Work out the finished part from the listing and answer in its coordinate system (mm). Face numbers are marked on the shaded views. Coordinates: 2 decimals unless noted, no trailing zeros. Order: outer loops, then holes, each group sorted by start corner. A loop starts at its lowest first (then second) coordinate and runs counter-clockwise, first axis right, second up. Notation, with made-up numbers: M 32,4 L 46,4 A21 ccw 46,31 Z; hole C -9,73.25 d10. An arc over 180 degrees is marked long. Answer in a Markdown table with one row per item. Add a question column.
Item 1: The part is cut by section A-A (z = 0). Write down the section's boundary in (x, y), then the cut area to 3 significant figures.
Item 2: The mould has two halves that part along Z. Classify the marked faces 1, 2 and 3: released by +Z, released by -Z, zero draft, split by the parting line, or undercut.
Item 3: Consider line 1 (Y direction, x = 5, z = 0); line 2 (Y direction, x = 2.25, z = -13.5); line 3 (Y direction, x = 5.75, z = 25). Determine where each line is inside the solid, lowest interval first. Write a range as from..to.
Item 4: Flat-ended cylindrical pins translate along their axes: pin 1 Ø3 at (x, y) = (1.5, 156) entering from -Z; pin 2 Ø2 at (x, z) = (7.5, 23) entering from +Y; pin 3 Ø5 at (x, y) = (2, -8.5) entering from +Z. Find the tip coordinate at first contact, or state that the pin passes through.
Item 5: The part is cut by section C-C (x = 2). Write down the section's boundary in (y, z).
Item 6: The part is cut by section B-B (y = 142.5). Write down the section's boundary in (x, z).
Item 7: The part is cut by section D-D (z = -20.5). Write down the section's boundary in (x, y), then the cut area to 3 significant figures.
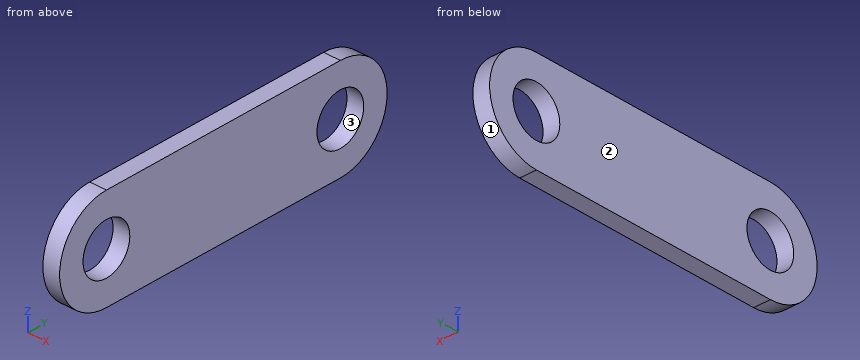
from build123d import *

# Parameters (mm, degrees)
SKETCH1_R           = 15
BOSS_EXTRUDE1_DEPTH = 10


with BuildPart() as part:
    # Sketch1 → Boss-Extrude1 (new body)
    with BuildSketch(Plane.YZ):
        with BuildLine():
            Line((0, 30), (150, 30))
            ThreePointArc((150, 30), (180, 0), (150, -30))
            Line((150, -30), (0, -30))
            ThreePointArc((0, -30), (-30, 0), (0, 30))
        make_face()
        with Locations(Location((0, 0, 0), (0, 0, 270))):
            Circle(SKETCH1_R, mode=Mode.SUBTRACT)
        with Locations(Location((150, 0, 0), (0, 0, 270))):
            Circle(SKETCH1_R, mode=Mode.SUBTRACT)
    extrude(amount=BOSS_EXTRUDE1_DEPTH)


solid = part.part
Reply:
| question | item | result |
|---|---|---|
| 1 | outline | M 0,-30 L 10,-30 L 10,-15 L 0,-15 Z; M 0,15 L 10,15 L 10,135 L 0,135 Z; M 0,165 L 10,165 L 10,180 L 0,180 Z |
| 1 | area | 1,500 mm2 |
| 2 | face 1 | split by the parting line |
| 2 | face 2 | zero draft |
| 2 | face 3 | undercut |
| 3 | line 1 | y = -30..-15, 15..135, 165..180 |
| 3 | line 2 | y = -26.79..-6.54, 6.54..143.46, 156.54..176.79 |
| 3 | line 3 | y = -16.58..166.58 |
| 4 | pin 1 | stops at z = -29.66 |
| 4 | pin 2 | stops at y = 170.4 |
| 4 | pin 3 | stops at z = 29.39 |
| 5 | outline | M 0,-30 L 150,-30 A30 ccw 150,30 L 0,30 A30 ccw Z; hole C 0,0 d30; hole C 150,0 d30 |
| 6 | outline | M 0,-30 L 10,-30 L 10,-12.99 L 0,-12.99 Z; M 0,12.99 L 10,12.99 L 10,30 L 0,30 Z |
| 7 | outline | M 0,-21.9 L 10,-21.9 L 10,171.9 L 0,171.9 Z |
| 7 | area | 1,940 mm2 |
